Design review of the part shown in the three views and the two pictorial views. Dimensions are in mm from the part's minimum x, y and z. A direction names the side the tool comes from. Coordinates: 2 decimals unless noted, no trailing zeros. Write each loop counter-clockwise with the first axis right and the second up, starting at its lowest first coordinate (ties: lowest second). Pieces come first, ordered by that corner, then holes. Notation, with made-up numbers: M 36.5,14.5 L 49.5,14.5 A7 ccw 49.5,22.5 Z; hole C 31.25,-28.75 d10. An arc over 180 degrees is marked long. Answer as a JSON object with one key per item and string values.
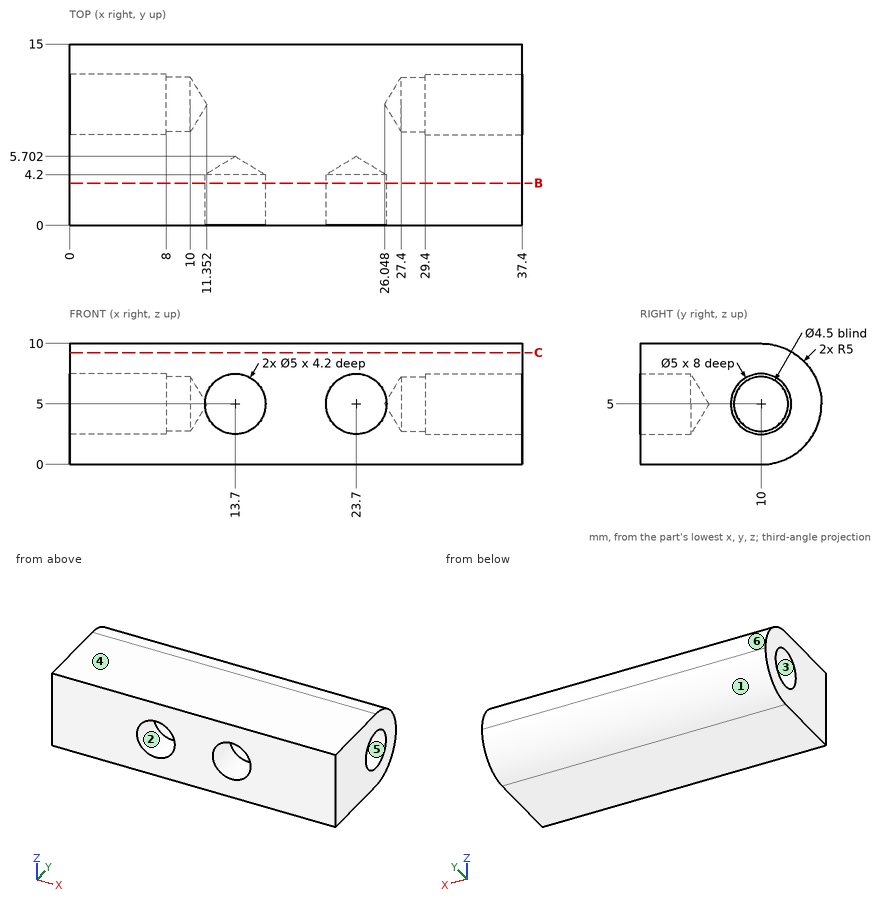
(1) Wall thickness on line 1 along Z through (x, y) = (9.6, 10); line 2 along X through (y, z) = (2, 6.75) (1 decimal); line 3 along Z through (x, y) = (33.75, 10): over which ranges is each line inside the solid? List them lowest first. Write a range as from..to.
Results list:
{"line 1": "0..2.75, 7.25..10", "line 2": "0..11.9, 15.5..21.9, 25.5..37.4", "line 3": "0..2.5, 7.5..10"}
(2) Add section B-B on y = 3.5. Give the boundary of the cut face in (x, z).
Results list:
{"outline": "M 0,0 L 37.4,0 L 37.4,10 L 0,10 Z; hole C 13.7,5 d5; hole C 23.7,5 d5"}
(3) Add section C-C on z = 9.25. Give the boundary of the cut face in (x, y), and give its area (4 significant figures).
Results list:
{"outline": "M 0,0 L 37.4,0 L 37.4,12.63 L 0,12.63 Z", "area": "472.5 mm²"}
(4) For the marked faces 1, 2 and 3, list the 3-axis set-ups (+Z, -Z, +X, -X, +Y, -Y) from which the entire face can be reached by the end or side of a thin tool; tool diameter is ignored.
Results list:
{"face 1": "-Z, +X, -X, +Y", "face 2": "-Y", "face 3": "-X"}
(5) For pin 1 Ø2.5 at (y, z) = (11, 4.5) entering from +X; pin 2 Ø2.5 at (y, z) = (10, 5) entering from -X; pin 3 Ø4 at (y, z) = (10, 5) entering from +X, all flat-tipped, find the tip position at first contact; note any pin that passes through.
Results list:
{"pin 1": "x = 29.4", "pin 2": "x = 10.6", "pin 3": "x = 27.25"}
(6) Draft analysis for pull direction Y (two halves, no side actions). For the marked faces 4, 5 and 6, state which applies: released by +Y, released by -Y, zero draft, split by the parting line, or undercut.
Results list:
{"face 4": "zero draft", "face 5": "undercut", "face 6": "released by +Y"}
